Read the model definition and answer for the solid it produces. Units are mm, in the model's axes. Give positions to 0.01 mm unless a question says otherwise; leave off trailing zeros. Order: outer loops, then holes, each group sorted by start corner. A loop starts at its lowest first (then second) coordinate and runs counter-clockwise, first axis right, second up. Notation, with made-up numbers: (87.25, 82.25) - (130.25, 82.25) arc R33 cw to (130.25, 114.25) - close; hole circle Ø2 at (-35, -38.5). An arc over 180 degrees is marked (long way). Return JSON: item names as keys, results as strings.
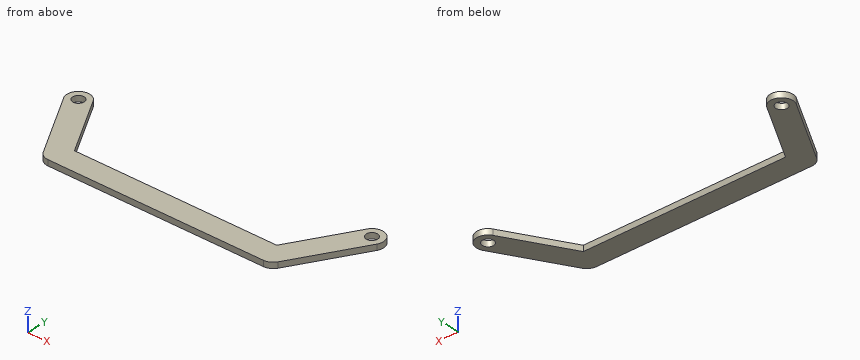
```python
from build123d import *

# Parameters (mm, degrees)
BOSS_EXTRUDE1_DEPTH = 31.75
SKETCH2_R           = 31.75
CUT_EXTRUDE1_DEPTH  = 995.439194974


with BuildPart() as part:
    # Sketch1 → Boss-Extrude1 (new body)
    with BuildSketch(Plane.XY):
        with BuildLine():
            Line((-605.529547439, 63.5), (605.529547439, 63.5))
            ThreePointArc((605.529547439, 63.5), (669.029547439, 0), (605.529547439, -63.5))
            Line((605.529547439, -63.5), (-605.529547439, -63.5))
            ThreePointArc((-605.529547439, -63.5), (-669.029547439, 0), (-605.529547439, 63.5))
        make_face()
        with BuildLine():
            Line((550.536934298, 31.75), (770.50738686, 412.75))
            ThreePointArc((770.50738686, 412.75), (857.25, 435.99261314), (880.49261314, 349.25))
            Line((880.49261314, 349.25), (660.522160579, -31.75))
            ThreePointArc((660.522160579, -31.75), (573.779547439, -54.99261314), (550.536934298, 31.75))
        make_face()
        with BuildLine():
            Line((-660.522160579, -31.75), (-880.49261314, 349.25))
            ThreePointArc((-880.49261314, 349.25), (-857.25, 435.99261314), (-770.50738686, 412.75))
            Line((-770.50738686, 412.75), (-550.536934298, 31.75))
            ThreePointArc((-550.536934298, 31.75), (-573.779547439, -54.99261314), (-660.522160579, -31.75))
        make_face()
    extrude(amount=-BOSS_EXTRUDE1_DEPTH)

    # Sketch2 → Cut-Extrude1 (cut, through all)
    with BuildSketch(Plane.XY):
        with Locations((825.5, 381)):
            Circle(SKETCH2_R)
        with Locations((-825.5, 381)):
            Circle(SKETCH2_R)
    extrude(amount=-CUT_EXTRUDE1_DEPTH, mode=Mode.SUBTRACT)


solid = part.part
```
Q1. A cutting plane is placed at B-B (y = 381). Write down the section's boundary in (x, z), and give its area (3 significant figures).
Values:
{"outline": "(-889, -31.75) - (-857.25, -31.75) - (-857.25, 0) - (-889, 0) - close; (-793.75, -31.75) - (-752.18, -31.75) - (-752.18, 0) - (-793.75, 0) - close; (752.18, -31.75) - (793.75, -31.75) - (793.75, 0) - (752.18, 0) - close; (857.25, -31.75) - (889, -31.75) - (889, 0) - (857.25, 0) - close", "area": "4,660 mm²"}
Q2. A cutting plane is placed at C-C (y = 230). Write down the section's boundary in (x, z), and give its area (3 significant figures).
Values:
{"outline": "(-811.64, -31.75) - (-665, -31.75) - (-665, 0) - (-811.64, 0) - close; (665, -31.75) - (811.64, -31.75) - (811.64, 0) - (665, 0) - close", "area": "9,310 mm²"}
Q3. Consider L1, parallel to X at y = 365, z = -11; L2, parallel to X at y = 368, z = -11; L3, parallel to Y at x = -502, z = -21. Determine where each line is inside the solid, lowest interval first.
Values:
{"L1": "x = -886.95 to -852.92, -798.08 to -742.94, 742.94 to 798.08, 852.92 to 886.95", "L2": "x = -887.66 to -854.47, -796.53 to -744.67, 744.67 to 796.53, 854.47 to 887.66", "L3": "y = -63.5 to 63.5"}
Q4. Given pin 1 (9.5 mm diameter, centred on x = 232.5, z = -18, fed in from +Y); pin 2 (2 mm diameter, centred on y = 299, z = -6.5, fed in from +X); pin 3 (8 mm diameter, centred on y = 378.5, z = -13.5, fed in from +X); pin 4 (12 mm diameter, centred on x = 423, y = 34, fed in from +Z), each flat-ended and moving along its own axis, determine where each tip first touches the part or whether it passes through.
Values:
{"pin 1": "stops at y = 63.5", "pin 2": "stops at x = 852.06", "pin 3": "stops at x = 889", "pin 4": "stops at z = 0"}
Q5. A cutting plane is placed at A-A (x = -825.5). Write down the section's boundary in (y, z), and give its area (3 significant figures).
Values:
{"outline": "(254, -31.75) - (349.25, -31.75) - (349.25, 0) - (254, 0) - close; (412.75, -31.75) - (444.5, -31.75) - (444.5, 0) - (412.75, 0) - close", "area": "4,030 mm²"}
Q6. A cutting plane is placed at D-D (x = -277). Write down the section's boundary in (y, z), and give its area (3 significant figures).
Values:
{"outline": "(-63.5, -31.75) - (63.5, -31.75) - (63.5, 0) - (-63.5, 0) - close", "area": "4,030 mm²"}
